Geometry: final body of the model. Coordinates: model frame, mm. Face numbers are marked on the shaded views. Round coordinates to 2 decimals unless told otherwise and drop trailing zeros. Write each loop counter-clockwise with the first axis right and the second up, starting at its lowest first coordinate (ties: lowest second). Pieces come first, ordered by that corner, then holes. Notation, with made-up numbers: (27, -22) -> (31, -22) arc R23 cw to (31, 10) -> close; hole circle Ø3 at (2, -3). An arc over 180 degrees is marked (long way). Use one line per item in the form item = value. Start each with the question number.
1. Cut plane B-B, the plane x = 2.5. Return the cut outline in (y, z).
2. Cut plane D-D, the plane y = 6.5. Return the cut outline in (x, z), plus the area to 3 significant figures.
3. Line query: L1, parallel to X at y = 4, z = 0; L2, parallel to Z at x = -3.5, y = 30; L3, parallel to Y at x = -5, z = -1.5. Output: solid intervals per line, ascending.
4. Cut plane C-C, the plane y = 37. Return the cut outline in (x, z).
5. Cut plane A-A, the plane x = -27. Return the cut outline in (y, z).
6. Draft query along Z for the marked faces 1, 2 and 3. Return one class per face: pulls with the +Z half, pulls with the -Z half, needs draft (parallel to the pull), parting line crosses it, or undercut.
7. Pin query (flat end, axial travel): pin 1 Ø17 at (y, z) = (23.5, -4.5) entering from +X; pin 2 Ø8 at (y, z) = (48, 1.5) entering from -X; pin 3 Ø16 at (x, z) = (27, 0) entering from +Y; pin 4 Ø11 at (x, z) = (-31.5, 11) entering from +Y. Return the tip coordinate at first contact, or that it passes through.
```python
from build123d import *
from build123d.topology import SkipClean

# Parameters (mm, degrees)
BOSS_EXTRUDE1_DEPTH      = 30
BOSS_EXTRUDE1_DEPTH_BACK = 30
SKETCH2_R                = 10
CUT_EXTRUDE1_DEPTH       = 5
BOSS_EXTRUDE2_START      = 3
SKETCH2_3_R              = 12
SKETCH2_3_R_2            = 10
BOSS_EXTRUDE2_DEPTH      = 3
SKETCH3_R                = 15
CUT_EXTRUDE2_DEPTH       = 8
BOSS_EXTRUDE3_START      = 3
SKETCH3_3_R              = 17
SKETCH3_3_R_2            = 15
BOSS_EXTRUDE3_DEPTH      = 3
FILLET1_R                = 15


with BuildPart() as part:
    # Sketch1 → Boss-Extrude1 (new, two sides: drawn at the far end of the back side and taken through both)
    with BuildSketch(Plane.XY.offset(-BOSS_EXTRUDE1_DEPTH_BACK)):
        with BuildLine():
            Line((50, 0), (-50, 0))
            Line((-50, 0), (-50, 5))
            Line((-50, 5), (-14, 5))
            ThreePointArc((-14, 5), (-6.928932188, 7.928932188), (-4, 15))
            Line((-4, 15), (-4, 55))
            Line((-4, 55), (4, 55))
            Line((4, 55), (4, 15))
            ThreePointArc((4, 15), (6.928932188, 7.928932188), (14, 5))
            Line((14, 5), (50, 5))
            Line((50, 5), (50, 0))
        make_face()
    extrude(amount=BOSS_EXTRUDE1_DEPTH + BOSS_EXTRUDE1_DEPTH_BACK)

    # Sketch2 → Cut-Extrude1 (cut)
    with BuildSketch(Plane(origin=(0, 5, 0), x_dir=(1, 0, 0), z_dir=(0, 1, 0))):
        with Locations(Location((-27, 0, 0), (0, 0, 270))):
            Circle(SKETCH2_R)
    cut_extrude1 = extrude(amount=-CUT_EXTRUDE1_DEPTH, mode=Mode.SUBTRACT)

    # Sketch2<3> → Boss-Extrude2 (add)
    with BuildSketch(Plane(origin=(0, 5, 0), x_dir=(1, 0, 0), z_dir=(0, 1, 0)).offset(BOSS_EXTRUDE2_START)):
        with Locations(Location((-27, 0, 0), (0, 0, 270))):
            Circle(SKETCH2_3_R)
        with Locations(Location((-27, 0, 0), (0, 0, 270))):
            Circle(SKETCH2_3_R_2, mode=Mode.SUBTRACT)
    boss_extrude2 = extrude(amount=-BOSS_EXTRUDE2_DEPTH)

    # Mirror1: Cut-Extrude1, Boss-Extrude2 across plane
    add(cut_extrude1.mirror(Plane(origin=(0, 0, 0), x_dir=(0, 0, 1), z_dir=(1, 0, 0))), mode=Mode.SUBTRACT)
    add(boss_extrude2.mirror(Plane(origin=(0, 0, 0), x_dir=(0, 0, 1), z_dir=(1, 0, 0))))

    # Sketch3 → Cut-Extrude2 (cut)
    with BuildSketch(Plane.ZY.offset(4)):
        with Locations(Location((0, 30, 0), (0, 0, 270))):
            Circle(SKETCH3_R)
    extrude(amount=-CUT_EXTRUDE2_DEPTH, mode=Mode.SUBTRACT)

    # Sketch3<3> → Boss-Extrude3 (add)
    with BuildSketch(Plane.ZY.offset(4).offset(BOSS_EXTRUDE3_START)):
        with Locations(Location((0, 30, 0), (0, 0, 241.927513064))):
            Circle(SKETCH3_3_R)
        with Locations((0, 30)):
            Circle(SKETCH3_3_R_2, mode=Mode.SUBTRACT)
    boss_extrude3 = extrude(amount=-BOSS_EXTRUDE3_DEPTH)

    # Mirror2: Boss-Extrude3 across plane
    with SkipClean():  # the faces are left unmerged after this step: merging them gives an invalid solid
        add(boss_extrude3.mirror(Plane(origin=(0, 0, 0), x_dir=(0, 0, 1), z_dir=(1, 0, 0))))

    # Fillet1
    fillet1_edges = [part.edges().sort_by_distance(p)[0] for p in [
        (0, 55, -30),
        (0, 55, 30),
    ]]
    fillet(fillet1_edges, radius=FILLET1_R)


solid = part.part
```
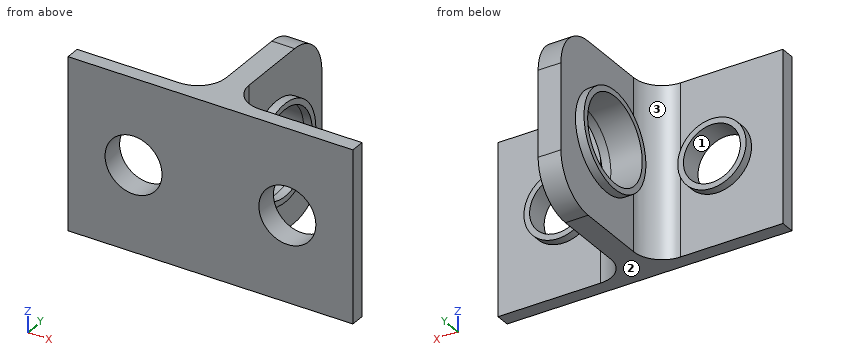
Outcome:
q1.outline = (0, -30) -> (40, -30) arc R15 ccw to (55, -15) -> (55, 15) arc R15 ccw to (40, 30) -> (0, 30) -> close; hole circle Ø30 at (30, 0)
q2.outline = circle Ø24 at (-27, 0); (-8.73, -30) -> (8.73, -30) -> (8.73, 30) -> (-8.73, 30) -> close; circle Ø24 at (27, 0); hole circle Ø20 at (-27, 0); hole circle Ø20 at (27, 0)
q2.area = 1,320 mm^2
q3.L1 = -50 to -37, -17 to 17, 37 to 50
q3.L2 = -30 to -15, 15 to 30
q3.L3 = 0 to 10.64, 13.07 to 15.08, 44.92 to 46.93
q4.outline = (-7, -15.49) -> (-4, -15.49) -> (-4, -30) -> (4, -30) -> (4, -15.49) -> (7, -15.49) -> (7, -13.27) -> (-7, -13.27) -> close; (-7, 13.27) -> (7, 13.27) -> (7, 15.49) -> (4, 15.49) -> (4, 30) -> (-4, 30) -> (-4, 15.49) -> (-7, 15.49) -> close
q5.outline = (0, -30) -> (5, -30) -> (5, -12) -> (8, -12) -> (8, -10) -> (0, -10) -> close; (0, 10) -> (8, 10) -> (8, 12) -> (5, 12) -> (5, 30) -> (0, 30) -> close
q6.face_1 = undercut
q6.face_2 = pulls with the -Z half
q6.face_3 = needs draft
q7.pin_1 = 7
q7.pin_2 = -7
q7.pin_3 = through
q7.pin_4 = 8
